from build123d import *

# Parameters (mm, degrees)
SKETCH1_W              = 30.48
SKETCH1_H              = 7.62
SKETCH1_R              = 2.286
BOSS_EXTRUDE1_DEPTH    = 2.54
FILLET1_R              = 2.54
FILLET2_R              = 5.08
CUT_EXTRUDE1_START     = -5.08
CUT_EXTRUDE1_OUTLINE_W = 5.08
CUT_EXTRUDE1_OUTLINE_H = 1.27
CUT_EXTRUDE1_DEPTH     = 5.08
FILLET3_R              = 0.635


# Read off the part's stored shape, not the designer's step: Cut-Extrude1
with BuildPart() as part:
    # Sketch1 → Boss-Extrude1 (new, symmetric)
    # profile 1 of 7: a face of its own
    with BuildSketch(Plane.XY):
        with Locations((2.54, 0)):
            Rectangle(SKETCH1_W, SKETCH1_H)
        Circle(SKETCH1_R, mode=Mode.SUBTRACT)
    # profile 2 of 7: a face of its own
    with BuildSketch(Plane.XY):
        with BuildLine():
            Line((-12.7, -16.51), (-12.7, -3.81))
            Line((-12.7, -3.81), (-12.7, 3.81))
            ThreePointArc((-12.7, 3.81), (-16.102954744, -8.89), (-12.7, -21.59))
            Line((-12.7, -21.59), (-12.7, -16.51))
        make_face()
    # profile 3 of 7: a face of its own
    with BuildSketch(Plane.XY):
        Polygon((-10.16, -3.81), (-12.7, -3.81), (-12.7, -16.51), (-10.16, -16.51), (-10.16, -8.89), align=None)
    # profile 4 of 7: a face of its own
    with BuildSketch(Plane.XY):
        Polygon((-10.16, -16.51), (-12.7, -16.51), (-12.7, -21.59), (10.16, -21.59), (10.16, -16.51), (9e-09, -16.51), align=None)
    # profile 5 of 7: a face of its own
    with BuildSketch(Plane.XY):
        with BuildLine():
            ThreePointArc((9e-09, -16.51), (-6.349999997, -14.393333336), (-10.16, -8.89))
            Line((-10.16, -8.89), (-10.16, -16.51))
            Line((-10.16, -16.51), (9e-09, -16.51))
        make_face()
    # profile 6 of 7: a face of its own
    with BuildSketch(Plane.XY):
        with BuildLine():
            ThreePointArc((10.16, -8.89), (6.350000003, -14.393333331), (9e-09, -16.51))
            Line((9e-09, -16.51), (10.16, -16.51))
            Line((10.16, -16.51), (10.16, -8.89))
        make_face()
    # profile 7 of 7: a face of its own
    with BuildSketch(Plane.XY):
        with BuildLine():
            ThreePointArc((10.16, -8.89), (6.350000003, -14.393333331), (9e-09, -16.51))
            Line((9e-09, -16.51), (10.16, -16.51))
            Line((10.16, -16.51), (10.16, -8.89))
        make_face()
    extrude(amount=BOSS_EXTRUDE1_DEPTH, both=True)

    # Fillet1
    fillet1_edges = [part.edges().sort_by_distance(p)[0] for p in [
        (10.16, -21.59, 0),
        (-12.7, -21.59, 0),
        (-12.7, 3.81, 0),
        (17.78, 3.81, 0),
        (17.78, -3.81, 0),
    ]]
    fillet(fillet1_edges, radius=FILLET1_R)

    # Fillet2
    fillet2_edges = [part.edges().sort_by_distance(p)[0] for p in [
        (-10.16, -3.81, 0),
    ]]
    fillet(fillet2_edges, radius=FILLET2_R - 0.0001)  # a hair under: the kernel refuses the full size

    # Cut-Extrude1 outline → Cut-Extrude1 (cut)
    with BuildSketch(Plane.XY.offset(2.54).offset(CUT_EXTRUDE1_START)):
        with BuildLine():
            ThreePointArc((-10.16, -8.89), (-8.672102448, -5.297897552), (-5.08, -3.81))
            Line((-5.08, -3.81), (-5.08, -2.54))
            Line((-5.08, -2.54), (-10.16, -2.54))
            Line((-10.16, -2.54), (-10.16, -8.89))
        make_face()
        with Locations((7.62, -3.175)):
            Rectangle(CUT_EXTRUDE1_OUTLINE_W, CUT_EXTRUDE1_OUTLINE_H)
        with Locations((7.62, 3.175)):
            Rectangle(CUT_EXTRUDE1_OUTLINE_W, CUT_EXTRUDE1_OUTLINE_H)
        with Locations((-7.62, 3.175)):
            Rectangle(CUT_EXTRUDE1_OUTLINE_W, CUT_EXTRUDE1_OUTLINE_H)
    extrude(amount=CUT_EXTRUDE1_DEPTH, mode=Mode.SUBTRACT)

    # Fillet3
    fillet3_edges = [part.edges().sort_by_distance(p)[0] for p in [
        (10.16, -8.89, 0),
    ]]
    fillet(fillet3_edges, radius=FILLET3_R)


solid = part.part
Could you check a few things on this model? Use its own coordinates, in mm. A direction names the side the tool comes from. Round coordinates to 2 decimals unless told otherwise and drop trailing zeros. Order: outer loops, then holes, each group sorted by start corner. A loop starts at its lowest first (then second) coordinate and runs counter-clockwise, first axis right, second up.
(1) Imagine slicing it at D-D (x = -5.5). Write out the boundary of the cut face in (y, z).
Response values:
outline: (-21.59, -2.54) - (-14.97, -2.54) - (-14.97, 2.54) - (-21.59, 2.54) - close; (-2.54, -2.54) - (2.54, -2.54) - (2.54, 2.54) - (-2.54, 2.54) - close
(2) I'm going to push flat-ended pins straight in: pin 1 (2 mm diameter, centred on x = -7, z = 0.5, fed in from +Y); pin 2 (3 mm diameter, centred on x = 9, y = -5.5, fed in from +Z); pin 3 (1.5 mm diameter, centred on x = 12.5, z = 0, fed in from -Y); pin 4 (2.5 mm diameter, centred on x = 8, z = -0.5, fed in from -Y). Where does each tip first touch, or does it pass through?
Response values:
pin 1: stops at y = 2.54
pin 2: passes through
pin 3: stops at y = -3.81
pin 4: stops at y = -21.59
(3) Imagine slicing it at B-B (y = 0). Write out the boundary of the cut face in (x, z), plus the area to 3 significant figures.
Response values:
outline: (-14.5, -2.54) - (-2.29, -2.54) - (-2.29, 2.54) - (-14.5, 2.54) - close; (2.29, -2.54) - (17.78, -2.54) - (17.78, 2.54) - (2.29, 2.54) - close
area: 141 mm2
(4) Please list where these lines run through material, in increasing order: line 1 along Y through (x, z) = (-5, -1.9); line 2 along Y through (x, z) = (9.5, -0.85); line 3 along X through (y, z) = (1, 1.65).
Response values:
line 1: y = -21.59 to -15.25, -3.81 to 3.81
line 2: y = -20.76 to -11.22, -2.54 to 2.54
line 3: x = -14.1 to -2.06, 2.06 to 17.78
(5) Imagine slicing it at A-A (x = 0). Write out the boundary of the cut face in (y, z), plus the area to 3 significant figures.
Response values:
outline: (-21.59, -2.54) - (-16.51, -2.54) - (-16.51, 2.54) - (-21.59, 2.54) - close; (-3.81, -2.54) - (-2.29, -2.54) - (-2.29, 2.54) - (-3.81, 2.54) - close; (2.29, -2.54) - (3.81, -2.54) - (3.81, 2.54) - (2.29, 2.54) - close
area: 41.3 mm2
(6) Which directions (+Z, -Z, +X, -X, +Y, -Y) give clear straight access to the entire face, cutting with the end or side of a thin tool? Please do faces 4 (the flat face through (-8, 2.54, 0)), 5 (the flat face through (0, -3.81, 0)), 6 (the flat face through (10.16, -3, 0)).
Response values:
face 4: +Z, -Z, +Y
face 5: +Z, -Z, +X
face 6: +Z, -Z
(7) If we mould it in two halves opening along X, with no side actions, what happens to faces 1 (the flat face through (-8, -2.54, 0)), 2 (the cylindrical face through (-12.5, -21.22, -0.04)), 3 (the flat face through (-3, -3, 2.54))? For each: released by +X, released by -X, zero draft, split by the parting line, or undercut.
Response values:
face 1: undercut
face 2: released by -X
face 3: zero draft
